Design review of the part built by this model. Coordinates are the model's own, in mm. A direction names the side the tool comes from. Round coordinates to 2 decimals unless told otherwise and drop trailing zeros. Write each loop counter-clockwise with the first axis right and the second up, starting at its lowest first coordinate (ties: lowest second). Pieces come first, ordered by that corner, then holes. Notation, with made-up numbers: M 14,83 L 46,83 A27 cw 46,118 Z; hole C -24.5,10.5 d11. An arc over 180 degrees is marked long. One line per question, with ' | ' between items. Start each with the question number.
Item 1: Machinability: for faces 1 (the face through (41, -13, 0)), 2 (the face through (40, -11, 0)), 3 (the face through (12, 0, 0)), which of the approach directions +Z, -Z, +X, -X, +Y, -Y give a long, thin tool a straight path to every point of the face, cutting with its end or side? Answer none if there is none.
Item 2: Insertion check: pin 1 Ø4 at (y, z) = (-7, -8.5) entering from +X; pin 2 Ø5 at (y, z) = (-5, 3.5) entering from -X; pin 3 Ø5 at (x, z) = (10, -6.5) entering from -Y. Each pin has a flat end and moves straight along its axis. Give the tip position at first contact, or say it passes through.
Item 3: Add section C-C, the plane z = 3. State the section outline as (x, y) points, and give its area (3 significant figures).
Item 4: For L1, parallel to Z at x = 10, y = 0.75; L2, parallel to Y at x = 33, z = 0; L3, parallel to X at y = -6.25, z = 0, list the stretches that pass through material, from the lowest coordinate up.
Item 5: Add section D-D, the plane y = 1.25. State the section outline as (x, z) points, and give its area (3 significant figures).
Item 6: Draft analysis for pull direction X (two halves, no side actions). For faces 4 (the face through (51.57, -12.01, 11)), 5 (the face through (1.5, 0.99, 11.07)), 6 (the face through (11.6, 1, -7.7)), state which applies: released by +X, released by -X, zero draft, split by the parting line, or undercut.
Item 7: Add section B-B, the plane x = 10. State the section outline as (y, z) points.
Item 8: Add section A-A, the plane z = -6.5. State the section outline as (x, y) points.
```python
from build123d import *

# Parameters (mm, degrees)
TABAN_FLAN_1_DEPTH    = 12.5
K_ELERI_START         = -13
K_ELERI_K_R1_DEPTH    = 15
IZIM2_R               = 2
KES_EKSTR_ZYON1_DEPTH = 10


# Read off the part's stored shape, not the designer's step: Köşeleri kır1
# Sheet-metal steps are written as plain solids
with BuildPart() as part:
    # Çizim1 → Taban-Flanş1 (new, symmetric)
    with BuildSketch(Plane.XY):
        with BuildLine():
            Line((53, -13), (27.7366, -13))
            ThreePointArc((27.7366, -13), (25.801531583, -12.198468417), (25, -10.2634))
            Line((25, -10.2634), (25, -0.7366))
            ThreePointArc((25, -0.7366), (24.784254855, -0.215745145), (24.2634, 0))
            Line((24.2634, 0), (0, 0))
            Line((0, 0), (0, 2))
            Line((0, 2), (24.2634, 2))
            ThreePointArc((24.2634, 2), (26.198468417, 1.198468417), (27, -0.7366))
            Line((27, -0.7366), (27, -10.2634))
            ThreePointArc((27, -10.2634), (27.215745145, -10.784254855), (27.7366, -11))
            Line((27.7366, -11), (53, -11))
            Line((53, -11), (53, -13))
        make_face()
    extrude(amount=TABAN_FLAN_1_DEPTH, both=True)

    # Köşeleri kır1 outline → Köşeleri kır1 (cut)
    with BuildSketch(Plane(origin=(0, 0, 0), x_dir=(1, 0, 0), z_dir=(0, 1, 0)).offset(K_ELERI_START)):
        with BuildLine():
            Line((53, 12.5), (48, 12.5))
            ThreePointArc((48, 12.5), (51.535533906, 11.035533906), (53, 7.5))
            Line((53, 7.5), (53, 12.5))
        make_face()
        with BuildLine():
            Line((53, -12.5), (53, -7.5))
            ThreePointArc((53, -7.5), (51.535533906, -11.035533906), (48, -12.5))
            Line((48, -12.5), (53, -12.5))
        make_face()
        with BuildLine():
            ThreePointArc((5, -12.5), (1.464466094, -11.035533906), (0, -7.5))
            Line((0, -7.5), (0, -12.5))
            Line((0, -12.5), (5, -12.5))
        make_face()
        with BuildLine():
            ThreePointArc((0, 7.5), (1.464466094, 11.035533906), (5, 12.5))
            Line((5, 12.5), (0, 12.5))
            Line((0, 12.5), (0, 7.5))
        make_face()
    extrude(amount=K_ELERI_K_R1_DEPTH, mode=Mode.SUBTRACT)

    # Çizim2 → Kes-Ekstrüzyon1 (cut)
    with BuildSketch(Plane(origin=(0, 2, 0), x_dir=(1, 0, 0), z_dir=(0, 1, 0))):
        with Locations(Location((10, 6.5, 0), (0, 0, 180))):
            Circle(IZIM2_R)
        with Locations((10, -6.5)):
            Circle(IZIM2_R)
    extrude(amount=-KES_EKSTR_ZYON1_DEPTH, mode=Mode.SUBTRACT)


solid = part.part
```
Computed values:
1) face 1: +Z, -Z, +X, -X, -Y | face 2: +Z, -Z, +X, +Y | face 3: +Z, -Z, -X, -Y
2) pin 1: stops at x = 27 | pin 2: stops at x = 25 | pin 3: stops at y = 0
3) outline: M 0,0 L 24.26,0 A0.74 cw 25,-0.74 L 25,-10.26 A2.74 ccw 27.74,-13 L 53,-13 L 53,-11 L 27.74,-11 A0.74 cw 27,-10.26 L 27,-0.74 A2.74 ccw 24.26,2 L 0,2 Z | area: 129 mm^2
4) L1: z = -12.5 to -8.5, -4.5 to 4.5, 8.5 to 12.5 | L2: y = -13 to -11 | L3: x = 25 to 27
5) outline: M 0,-7.5 A5 ccw 5,-12.5 L 26.15,-12.5 L 26.15,12.5 L 5,12.5 A5 ccw 0,7.5 Z; hole C 10,-6.5 d4; hole C 10,6.5 d4 | area: 618 mm^2
6) face 4: released by +X | face 5: released by -X | face 6: undercut
7) outline: M 0,-12.5 L 2,-12.5 L 2,-8.5 L 0,-8.5 Z; M 0,-4.5 L 2,-4.5 L 2,4.5 L 0,4.5 Z; M 0,8.5 L 2,8.5 L 2,12.5 L 0,12.5 Z
8) outline: M 0,0 L 8,0 L 8,2 L 0,2 Z; M 12,0 L 24.26,0 A0.74 cw 25,-0.74 L 25,-10.26 A2.74 ccw 27.74,-13 L 53,-13 L 53,-11 L 27.74,-11 A0.74 cw 27,-10.26 L 27,-0.74 A2.74 ccw 24.26,2 L 12,2 Z
